Source: CAD feature listing. Evaluate the final solid. Frame: model axes, mm. Face numbers are marked on the shaded views. A direction names the side the tool comes from. Give positions to 0.01 mm unless a question says otherwise; leave off trailing zeros. Order: outer loops, then holes, each group sorted by start corner. A loop starts at its lowest first (then second) coordinate and runs counter-clockwise, first axis right, second up. Notation, with made-up numbers: M 87,-12 L 132,-12 A20 ccw 132,11 Z; hole C 86.5,63 d1. An arc over 180 degrees is marked long. Use CSV: the item, a comma, the result in double quotes. Start each with the question number.
1. Line query: line 1 along Z through (x, y) = (0, 5.5); line 2 along X through (y, z) = (5.75, 0) (3 decimals); line 3 along X through (y, z) = (3.75, 1.25). Output: solid intervals per line, ascending. Write a range as [from, to].
2. Section query D-D, the plane y = -3.5. Return the cut outline in (x, z).
3. Pin query (flat end, axial travel): P1, Ø1, axis at x = -2, y = 1, coming from the +Z side; P2, Ø2, axis at x = -3, z = -3.5, coming from the -Y side; P3, Ø3, axis at y = 1, z = 3, coming from the +X side; P4, Ø1, axis at y = -3.5, z = 3.5, coming from the +X side. Return the tip coordinate at first contact, or that it passes through.
4. Section query C-C, the plane z = 0. Return the cut outline in (x, y) (3 decimals).
5. Section query A-A, the plane y = 3.5. Return the cut outline in (x, z) (3 decimals), plus the area to 3 significant figures.
6. Mould query, pull axis X, two halves, no side actions, for the marked faces 4, 5, 6 and 7. Classes: released by +X, released by -X, zero draft, split by the parting line, or undercut.
7. Reachability of the marked faces 1, 2 and 3 from +Z, -Z, +X, -X, +Y, -Y: full face, straight path, thin tool, end or side. Return the list, or none.
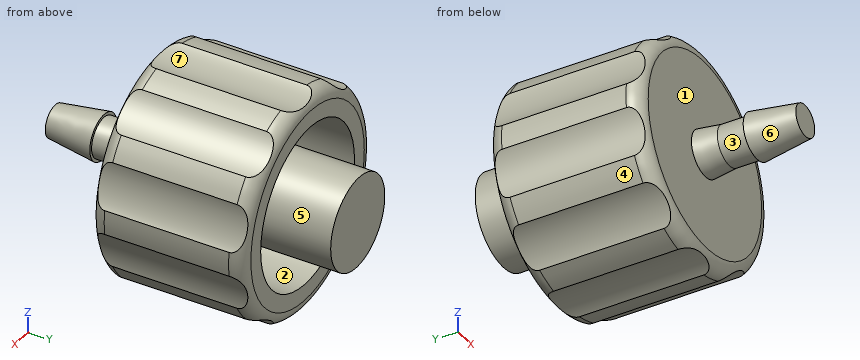
from build123d import *

# Parameters (mm, degrees)
SKETCH1_R           = 5.535
BOSS_EXTRUDE1_DEPTH = 7.6
FILLET1_R           = 0.7
SKETCH2_R           = 3
CUT_EXTRUDE1_DEPTH  = 7.6
CIRPATTERN1_COUNT   = 10
SKETCH4_R           = 4
CUT_EXTRUDE2_DEPTH  = 6.4
SKETCH5_R           = 2.307777858
BOSS_EXTRUDE2_DEPTH = 8.9


with BuildPart() as part:
    # Sketch1 → Boss-Extrude1 (new body)
    with BuildSketch(Plane(origin=(0, 0, 0), x_dir=(1, 0, 0), z_dir=(0, 1, 0))):
        Circle(SKETCH1_R)
    extrude(amount=BOSS_EXTRUDE1_DEPTH)

    # Fillet1
    fillet1_edges = [part.edges().sort_by_distance(p)[0] for p in [
        (-5.535, 0, 0),
        (-5.535, 7.6, 0),
    ]]
    fillet(fillet1_edges, radius=FILLET1_R)

    # Sketch2 → Cut-Extrude1 (cut)
    with BuildSketch(Plane(origin=(0, 0, 0), x_dir=(-1, 0, 0), z_dir=(0, -1, 0))):
        with Locations((0, 8.212488156)):
            Circle(SKETCH2_R)
    cut_extrude1 = extrude(amount=-CUT_EXTRUDE1_DEPTH, mode=Mode.SUBTRACT)

    # CirPattern1: Cut-Extrude1 ×10 about axis
    cirpattern1_axis = Axis((0, 0, 0), (0, 1, 0))
    for i in range(1, CIRPATTERN1_COUNT):
        add(cut_extrude1.rotate(cirpattern1_axis, i * 360 / CIRPATTERN1_COUNT), mode=Mode.SUBTRACT)

    # Sketch3 → Revolve1 (revolve)
    with BuildSketch(Plane.XY):
        Polygon((1.15, 0), (1, -1.2), (1, -2.58), (1.15, -2.58), (0.81, -5), (0, -5), (0, 0), align=None)
    revolve(axis=Axis((0, -5, 0), (0, 1, 0)))

    # Sketch4 → Cut-Extrude2 (cut)
    with BuildSketch(Plane(origin=(0, 7.6, 0), x_dir=(1, 0, 0), z_dir=(0, 1, 0))):
        Circle(SKETCH4_R)
    extrude(amount=-CUT_EXTRUDE2_DEPTH, mode=Mode.SUBTRACT)

    # Sketch5 → Boss-Extrude2 (add)
    with BuildSketch(Plane(origin=(0, 1.2, 0), x_dir=(1, 0, 0), z_dir=(0, 1, 0))):
        Circle(SKETCH5_R)
    extrude(amount=BOSS_EXTRUDE2_DEPTH)


solid = part.part
Result set:
1,line 1,"[-5.21, -4], [-2.31, 2.31], [4, 5.21]"
1,line 2,"[-5.535, -4], [-2.308, 2.308], [4, 5.535]"
1,line 3,"[-5.1, -3.8], [-1.94, 1.94], [3.8, 5.1]"
2,outline,"C 0,0 d2.04"
3,P1,"z = 5.33"
3,P2,"y = 0"
3,P3,"x = 5"
3,P4,"through"
4,outline,"M -5.535,0.7 A0.7 ccw -4.835,0 L -1.15,0 L -1,-1.2 L -1,-2.58 L -1.15,-2.58 L -0.81,-5 L 0.81,-5 L 1.15,-2.58 L 1,-2.58 L 1,-1.2 L 1.15,0 L 4.835,0 A0.7 ccw 5.535,0.7 L 5.535,6.9 A0.7 ccw 4.835,7.6 L 4,7.6 L 4,1.2 L 2.308,1.2 L 2.308,10.1 L -2.308,10.1 L -2.308,1.2 L -4,1.2 L -4,7.6 L -4.835,7.6 A0.7 ccw -5.535,6.9 Z"
5,outline,"M -5.5,-0.625 A3 cw -4.817,-2.727 A5.535 ccw -4.082,-3.738 A3 cw -2.294,-5.037 A5.535 ccw -1.105,-5.424 A3 cw 1.105,-5.424 A5.535 ccw 2.294,-5.037 A3 cw 4.082,-3.738 A5.535 ccw 4.817,-2.727 A3 cw 5.5,-0.625 A5.535 ccw 5.5,0.625 A3 cw 4.817,2.727 A5.535 ccw 4.082,3.738 A3 cw 2.294,5.037 A5.535 ccw 1.105,5.424 A3 cw -1.105,5.424 A5.535 ccw -2.294,5.037 A3 cw -4.082,3.738 A5.535 ccw -4.817,2.727 A3 cw -5.5,0.625 A5.535 ccw Z; C 0,0 d4.616; hole C 0,0 d8"
5,area,"57.9 mm2"
6,face 4,"released by -X"
6,face 5,"undercut"
6,face 6,"split by the parting line"
6,face 7,"undercut"
7,face 1,"-Y"
7,face 2,"+Y"
7,face 3,"none"
